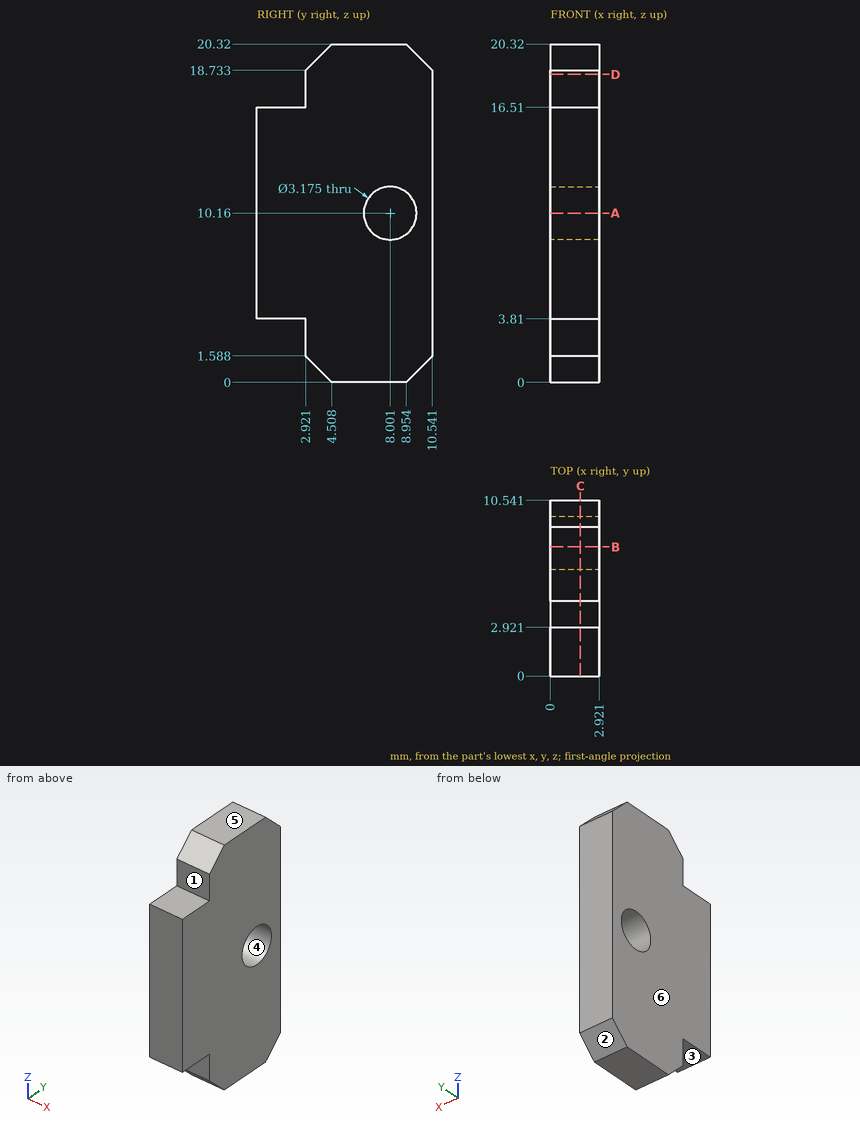
Study the drawing (mm; zero at the part's minimum x, y, z) and answer. A direction names the side the tool comes from. Round coordinates to 2 decimals unless told otherwise and drop trailing zeros. Loops run counter-clockwise (first coordinate to the right, second up) from the corner with the lowest first, then second, coordinate; pieces in that order, holes last.
Q1. Which of the six approach directions +Z, -Z, +X, -X, +Y, -Y give full straight-line access (tool end or side, diameter ignored) to the marked faces 1, 2 and 3?
Q2. For a pull along Z with two mould halves and no side action, classify the marked faces 4, 5 and 6 as released by +Z, released by -Z, zero draft, split by the parting line, or undercut.
Q3. Section B-B, the plane y = 7.75 is taken. Determine the outline of the cut face in (x, z), then the cut area to 3 significant figures.
Q4. Section C-C, the plane x = 1.8 is taken. Determine the outline of the cut face in (y, z) (1 decimal).
Q5. Find the intervals of material crossed by line 1 (Y direction, x = 2.15, z = 10.16); line 2 (Z direction, x = 1.8, y = 0.5); line 3 (Y direction, x = 0.4, z = 10.5), in increasing order.
Q6. Section D-D, the plane z = 18.5 is taken. Determine the outline of the cut face in (x, y).
Q7. Section A-A, the plane z = 10.16 is taken. Determine the outline of the cut face in (x, y).
Q8. Given pin 1 Ø0.9 at (x, y) = (0.5, 2) entering from +Z; pin 2 Ø1.1 at (x, z) = (2, 2.5) entering from -Y; pin 3 Ø1.5 at (x, y) = (1.5, 2) entering from -Z, each flat-ended and moving along its own axis, determine where each tip first touches the part or whether it passes through.
Completed:
1. face 1: +Z, +X, -X, -Y
1. face 2: -Z, +X, -X, +Y
1. face 3: -Z, +X, -X, -Y
2. face 4: undercut
2. face 5: released by +Z
2. face 6: zero draft
3. outline: (0, 0) - (2.92, 0) - (2.92, 8.59) - (0, 8.59) - close; (0, 11.73) - (2.92, 11.73) - (2.92, 20.32) - (0, 20.32) - close
3. area: 50.2 mm2
4. outline: (0, 3.8) - (2.9, 3.8) - (2.9, 1.6) - (4.5, 0) - (9, 0) - (10.5, 1.6) - (10.5, 18.7) - (9, 20.3) - (4.5, 20.3) - (2.9, 18.7) - (2.9, 16.5) - (0, 16.5) - close; hole circle Ø3.2 at (8, 10.2)
5. line 1: y = 0 to 6.41, 9.59 to 10.54
5. line 2: z = 3.81 to 16.51
5. line 3: y = 0 to 6.45, 9.55 to 10.54
6. outline: (0, 2.92) - (2.92, 2.92) - (2.92, 10.54) - (0, 10.54) - close
7. outline: (0, 0) - (2.92, 0) - (2.92, 6.41) - (0, 6.41) - close; (0, 9.59) - (2.92, 9.59) - (2.92, 10.54) - (0, 10.54) - close
8. pin 1: stops at z = 16.51
8. pin 2: stops at y = 2.92
8. pin 3: stops at z = 3.81
